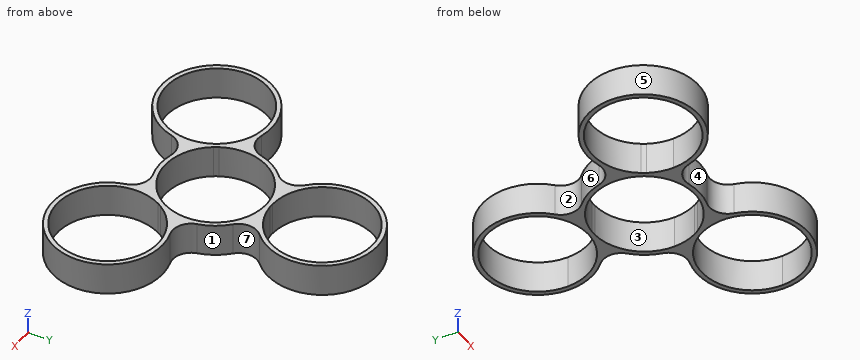
```python
from build123d import *

# Parameters (mm, degrees)
F1_DEPTH = 7


with BuildPart() as f1:
    # F0 (on Top) → F1 (new body)
    with BuildSketch(Plane.XY):
        with BuildLine():
            ThreePointArc((8.343223, 8.625), (7.124298, 11.5), (8.343223, 14.375))
            ThreePointArc((8.343223, 14.375), (0, 35), (-8.343223, 14.375))
            ThreePointArc((-8.343223, 14.375), (-7.124298, 11.5), (-8.343223, 8.625))
            ThreePointArc((-8.343223, 8.625), (-10.392305, 6), (-11.641081, 2.912943))
            ThreePointArc((-11.641081, 2.912943), (-13.521441, 0.419823), (-16.620727, 0.037943))
            ThreePointArc((-16.620727, 0.037943), (-30.310889, -17.5), (-8.277504, -14.412943))
            ThreePointArc((-8.277504, -14.412943), (-6.397143, -11.919823), (-3.297857, -11.537943))
            ThreePointArc((-3.297857, -11.537943), (0, -12), (3.297857, -11.537943))
            ThreePointArc((3.297857, -11.537943), (6.397143, -11.919823), (8.277504, -14.412943))
            ThreePointArc((8.277504, -14.412943), (30.310889, -17.5), (16.620727, 0.037943))
            ThreePointArc((16.620727, 0.037943), (13.521441, 0.419823), (11.641081, 2.912943))
            ThreePointArc((11.641081, 2.912943), (10.392305, 6), (8.343223, 8.625))
        make_face()
        with BuildLine():
            ThreePointArc((-10.114012, -6.458078), (-9.203034, -8.906237), (-8.893584, -11.5))
            ThreePointArc((-8.893584, -11.5), (-30.495404, -14.611511), (-10.649865, -5.529952))
            ThreePointArc((-10.649865, -5.529952), (-10.370654, -5.9875), (-10.114012, -6.458078))
        make_face(mode=Mode.SUBTRACT)
        with BuildLine():
            ThreePointArc((10.649865, -5.529952), (23.030095, -0.92318), (30.943584, -11.5))
            ThreePointArc((30.943584, -11.5), (17.324822, -22.21555), (10.114012, -6.458078))
            ThreePointArc((10.114012, -6.458078), (10.370654, -5.9875), (10.649865, -5.529952))
        make_face(mode=Mode.SUBTRACT)
        with BuildLine():
            ThreePointArc((0.535854, 11.01197), (7.983057, 7.60404), (11.025, 0))
            ThreePointArc((11.025, 0), (10.71555, -2.593763), (9.804573, -5.041922))
            ThreePointArc((9.804573, -5.041922), (9.54793, -5.5125), (9.268719, -5.970048))
            ThreePointArc((9.268719, -5.970048), (0, -11.025), (-9.268719, -5.970048))
            ThreePointArc((-9.268719, -5.970048), (-9.54793, -5.5125), (-9.804573, -5.041922))
            ThreePointArc((-9.804573, -5.041922), (-9.54793, 5.5125), (-0.535854, 11.01197))
            ThreePointArc((-0.535854, 11.01197), (0, 11.025), (0.535854, 11.01197))
        make_face(mode=Mode.SUBTRACT)
        with BuildLine():
            ThreePointArc((-0.535854, 11.98803), (-7.60404, 30.983057), (11.025, 23))
            ThreePointArc((11.025, 23), (7.983057, 15.39596), (0.535854, 11.98803))
            ThreePointArc((0.535854, 11.98803), (0, 11.975), (-0.535854, 11.98803))
        make_face(mode=Mode.SUBTRACT)
    extrude(amount=F1_DEPTH)


solid = f1.part
```
Check sheet for the modelled part. Datum: model origin and axes. Units: mm. Face numbers are marked on the shaded views. A direction names the side the tool comes from. Round coordinates to 2 decimals unless told otherwise and drop trailing zeros. Loops run counter-clockwise (first coordinate to the right, second up) from the corner with the lowest first, then second, coordinate; pieces in that order, holes last. Notation, with made-up numbers: (89, 30) - (128, 30) arc R7 ccw to (128, 42) - close; hole circle Ø3 at (-3.5, 53.25). An arc over 180 degrees is marked (long way). Answer as a JSON object with one key per item and string values. Group by question number.
Q1. Gauge pin test, flat ends, axial feed: P1, Ø2, axis at x = 16, z = 5.5, coming from the -Y side; P2, Ø2, axis at y = 18.5, z = 5.5, coming from the -X side. Record the tip position at first contact, or that the pin passes through.
Q2. Sectioned sample at B-B, the plane x = -17.5. Enter the section's corners in (y, z).
Q3. Sectioned sample at C-C, the plane y = -8.5. Enter the section's corners in (x, z), plus the area to 3 significant figures.
Q4. Sectioned sample at D-D, the plane z = 3. Count the separate pieces of the cut face and the enclosed holes in it, plus the area to 3 significant figures.
Q5. Sectioned sample at A-A, the plane y = 5.5. Enter the section's corners in (x, z).
Q6. Mould release check, pull along X, two halves, no side actions. Record for the marked faces 4, 5, 6 and 7: released by +X, released by -X, zero draft, split by the parting line, or undercut.
Q7. Set-up check for the marked faces 1, 2 and 3: record each of +Z, -Z, +X, -X, +Y, -Y from which the full face is reachable in a straight line by a thin tool's end or side.
Q8. Scan lines: line 1 along Y through (x, z) = (-0.5, 4); line 2 along X through (y, z) = (23, 5.5) (3 decimals); line 3 along X through (y, z) = (-3.5, 4.25). Record each from-to range of solid material in increasing order. Write a range as [from, to].
Solution:
{
 "1": {"P1": "stops at y = -23.14", "P2": "stops at x = -11.48"},
 "2": {"outline": "(-23.25, 0) - (-22.26, 0) - (-22.26, 7) - (-23.25, 7) - close; (-0.74, 0) - (0.25, 0) - (0.25, 7) - (-0.74, 7) - close"},
 "3": {"outline": "(-31.54, 0) - (-30.53, 0) - (-30.53, 7) - (-31.54, 7) - close; (-9.31, 0) - (-7.02, 0) - (-7.02, 7) - (-9.31, 7) - close; (7.02, 0) - (9.31, 0) - (9.31, 7) - (7.02, 7) - close; (30.53, 0) - (31.54, 0) - (31.54, 7) - (30.53, 7) - close", "area": "46.2 mm²"},
 "4": {"separate pieces": "1", "enclosed holes": "4", "area": "308 mm²"},
 "5": {"outline": "(-10.67, 0) - (-9.56, 0) - (-9.56, 7) - (-10.67, 7) - close; (9.56, 0) - (10.67, 0) - (10.67, 7) - (9.56, 7) - close"},
 "6": {"face 4": "undercut", "face 5": "undercut", "face 6": "released by -X", "face 7": "released by +X"},
 "7": {"face 1": "+Z, -Z, +X", "face 2": "+Z, -Z, -X", "face 3": "+Z, -Z"},
 "8": {"line 1": "y = [-11.99, -11.01], [11.01, 11.99], [34.01, 34.99]", "line 2": "x = [-12, -11.025], [11.025, 12]", "line 3": "x = [-28.86, -27.5], [-12.33, -10.45], [10.45, 12.33], [27.5, 28.86]"}
}
